Read the model definition and answer for the solid it produces. Units are mm, in the model's axes. A direction names the side the tool comes from. Give positions to 0.01 mm unless a question says otherwise; leave off trailing zeros. Loops run counter-clockwise (first coordinate to the right, second up) from the corner with the lowest first, then second, coordinate; pieces in that order, holes last. Notation, with made-up numbers: (41, 82) - (70, 82) arc R14 ccw to (70, 87) - close; hole circle Ø10 at (12.5, 52.25). An arc over 180 degrees is marked (long way). Write item = value, one per line. Start each with the question number.
from build123d import *

# Parameters (mm, degrees)
F0_W     = 126
F0_H     = 124
F0_W_2   = 11
F0_W_3   = 3
F1_DEPTH = 5
F2_DEPTH = 9
F3_R     = 60
F3_R_2   = 7.5
F4_DEPTH = 2
F5_R     = 1
F6_DEPTH = 2
F7_R     = 1
F8_DEPTH = 1


# Not quite as in the source:
# - a feature names something its author has since deleted; it is built from what else it names


with BuildPart() as f1:
    # F0 (on Top) → F1 (new body)
    with BuildSketch(Plane.XY):
        with Locations((4, 0)):
            Rectangle(F0_W, F0_H)
        with Locations((-64.5, 0)):
            Rectangle(F0_W_2, F0_H)
        with Locations((68.5, 0)):
            Rectangle(F0_W_3, F0_H)
    extrude(amount=F1_DEPTH)

    # F0 (on Top) → F2 (join)
    with BuildSketch(Plane.XY):
        with Locations((-64.5, 0)):
            Rectangle(F0_W_2, F0_H)
        with Locations((68.5, 0)):
            Rectangle(F0_W_3, F0_H)
    extrude(amount=F2_DEPTH)

    # F3 (on face) → F4 (cut)
    with BuildSketch(Plane.XY.offset(5)):
        with Locations((6.0000000522, 0)):
            Circle(F3_R)
        with Locations((6.0000000522, 0)):
            Circle(F3_R_2, mode=Mode.SUBTRACT)
    extrude(amount=-F4_DEPTH, mode=Mode.SUBTRACT)

    # F5 (on face) → F6 (cut)
    with BuildSketch(Plane.XY.offset(5)):
        with Locations((6.0000000522, 0)):
            Circle(F5_R)
    extrude(amount=-F6_DEPTH, mode=Mode.SUBTRACT)

    # F7 (on face) → F8 (cut)
    with BuildSketch(Plane.XZ.offset(62)):
        with Locations((-64.9999976158, 4)):
            Circle(F7_R)
    extrude(amount=-F8_DEPTH, mode=Mode.SUBTRACT)


solid = f1.part
1. Given P1, Ø1.8, axis at x = -65, z = 4, coming from the -Y side; P2, Ø1, axis at x = -6.5, y = 25, coming from the +Z side; P3, Ø5, axis at x = 13.5, y = 4.5, coming from the +Z side, each flat-ended and moving along its own axis, determine where each tip first touches the part or whether it passes through.
2. A cutting plane is placed at D-D on x = 61. Give the vertices of the cut face in (y, z).
3. A cutting plane is placed at A-A on z = 6.75. Give the vertices of the cut face in (x, y).
4. A cutting plane is placed at C-C on x = -34. Give the vertices of the cut face in (y, z).
5. For a pull along Y with two mould halves and no side action, classify faces 1 (the cylindrical face through (63.23, 18.02, 4.01)), 2 (the flat face through (1, 62, 2)), 3 (the flat face through (-59, -1, 7)) as released by +Y, released by -Y, zero draft, split by the parting line, or undercut.
6. A tool of negligible diameter and unlimited length cuts with its end or side. For faces 4 (the flat face through (68, 1, 9)), 5 (the flat face through (6, -2, 5)), 6 (the flat face through (5, -12, 3)), from which of +Z, -Z, +X, -X, +Y, -Y can it reach the whole face along a straight path? Write none if from no direction.
7. Consider line 1 along Y through (x, z) = (6, 4); line 2 along X through (y, z) = (-1.5, 8.5); line 3 along X through (y, z) = (-6.5, 4.75). Determine where each line is inside the solid, lowest interval first. Write a range as [from, to].
8. A cutting plane is placed at B-B on y = 14.5. Give the vertices of the cut face in (x, z), and give its area (3 significant figures).
Reply:
q1.P1 = -61
q1.P2 = 3
q1.P3 = 5
q2.outline = (-62, 0) - (62, 0) - (62, 5) - (23.98, 5) - (23.98, 3) - (-23.98, 3) - (-23.98, 5) - (-62, 5) - close
q3.outline = (-70, -62) - (-59, -62) - (-59, 62) - (-70, 62) - close; (67, -62) - (70, -62) - (70, 62) - (67, 62) - close
q4.outline = (-62, 0) - (62, 0) - (62, 5) - (44.72, 5) - (44.72, 3) - (-44.72, 3) - (-44.72, 5) - (-62, 5) - close
q5.face_1 = undercut
q5.face_2 = released by +Y
q5.face_3 = zero draft
q6.face_4 = +Z, +X, -X, +Y, -Y
q6.face_5 = +Z, +Y, -Y
q6.face_6 = +Z
q7.line_1 = [-62, -60], [-7.5, -1], [1, 7.5], [60, 62]
q7.line_2 = [-70, -59], [67, 70]
q7.line_3 = [-70, -53.65], [2.26, 9.74], [65.65, 70]
q8.outline = (-70, 0) - (70, 0) - (70, 9) - (67, 9) - (67, 5) - (64.22, 5) - (64.22, 3) - (-52.22, 3) - (-52.22, 5) - (-59, 5) - (-59, 9) - (-70, 9) - close
q8.area = 523 mm^2
